```python
from build123d import *

# Parameters (mm, degrees)
BOSS_EXTRUDE1_DEPTH       = 12.7
SKETCH2_R                 = 5.635000033
HAPTIC_MOTOR_CUTOUT_DEPTH = 9.557999934
SKETCH3_W                 = 5.08
SKETCH3_H                 = 6.35
HAPTIC_WIRE_CUTOUT_DEPTH  = 13.7
SKETCH4_W                 = 6.096
SKETCH4_H                 = 2.54
PINS_DEPTH                = 5.08


with BuildPart() as part:
    # Sketch1 → Boss-Extrude1 (new body)
    with BuildSketch(Plane(origin=(0, 0, 0), x_dir=(1, 0, 0), z_dir=(0, 1, 0))):
        Polygon((0, 0), (19.05, 0), (12.7, 19.05), (19.05, 38.1), (0, 38.1), (-6.35, 19.05), align=None)
    extrude(amount=BOSS_EXTRUDE1_DEPTH)

    # Sketch2 → Haptic Motor Cutout (cut)
    with BuildSketch(Plane.XZ.offset(-12.7)):
        with Locations((2.54, -19.05)):
            Circle(SKETCH2_R)
    extrude(amount=HAPTIC_MOTOR_CUTOUT_DEPTH, mode=Mode.SUBTRACT)

    # Sketch3 → Haptic Wire Cutout (cut, through all)
    with BuildSketch(Plane.XZ):
        with Locations((2.54, -27.255072104)):
            Rectangle(SKETCH3_W, SKETCH3_H)
    extrude(amount=-HAPTIC_WIRE_CUTOUT_DEPTH, mode=Mode.SUBTRACT)

    # Sketch4 → Pins (add)
    with BuildSketch(Plane.XZ):
        with Locations((10.668, -35.56)):
            Rectangle(SKETCH4_W, SKETCH4_H)
    pins = extrude(amount=PINS_DEPTH)

    # Mirror1: Pins across plane
    add(pins.mirror(Plane(origin=(0, 0, -19.05), x_dir=(1, 0, 0), z_dir=(0, 0, -1))))


solid = part.part
```
Can you work these out from the model? Positions are in its coordinate system, mm. A direction names the side the tool comes from. Coordinates: 2 decimals unless noted, no trailing zeros. Loops run counter-clockwise (first coordinate to the right, second up) from the corner with the lowest first, then second, coordinate; pieces in that order, holes last.
1) Thinking about a two-plate mould opening in Z: for faces 6 (the flat face through (15.83, 6.26, -28.44)), 7 (the flat face through (9, 6, 0)), 8 (the flat face through (13.716, -3, -36)), which applies, pulls with the +Z half, pulls with the -Z half, needs draft (parallel to the pull), parting line crosses it, or undercut?
2) For pin 1 (4 mm diameter, centred on y = 0, z = -6.5, fed in from -X); pin 2 (2 mm diameter, centred on x = -2.5, z = -23, fed in from -Y); pin 3 (8.5 mm diameter, centred on x = 3.5, z = -20, fed in from +Y); pin 4 (5 mm diameter, centred on y = 9, z = -19.5, fed in from -X), each with a flat end and sliding along its axis, tell me the tip position at first contact or that it passes through.
3) Which directions (+Z, -Z, +X, -X, +Y, -Y) give clear straight access to the entire face, cutting with the end or side of a thin tool? Please do faces 1 (the flat face through (11, -3, -3.81)), 2 (the flat face through (11, -3, -36.83)), 3 (the flat face through (11, -3, -1.27)), 4 (the flat face through (5.08, 6, -27)), 5 (the flat face through (7.62, -3, -3)).
4) Imagine slicing it at B-B on y = 6. List the corners of the cut face in (x, z) for me (3 decimals), plus the area to 3 significant figures.
5) Imagine slicing it at C-C on y = -1.75. List the corners of the cut face in (x, z) for me, plus the area to 3 significant figures.
6) Imagine slicing it at D-D on x = 11.5. List the corners of the cut face in (y, z) for me, plus the area to 3 significant figures.
7) Imagine slicing it at A-A on x = 2.54. List the corners of the cut face in (y, z) for me (3 decimals), plus the area to 3 significant figures.
8) I need wall thicknesses on probe 1 along Z at (x, y) = (2.54, 10) (3 decimals); probe 2 along X at (y, z) = (10.75, -19.05) (3 decimals); probe 3 along Y at (x, z) = (14.5, -35). Which ranges of each line are inside material? Lowest first, please.
Completed:
1. face 6: undercut
1. face 7: pulls with the +Z half
1. face 8: needs draft
2. pin 1: stops at x = -2.83
2. pin 2: stops at y = 0
2. pin 3: stops at y = 3.14
2. pin 4: stops at x = -6.35
3. face 1: +X, -X, -Y
3. face 2: -Z, +X, -X, -Y
3. face 3: +Z, +X, -X, -Y
3. face 4: +Y, -Y
3. face 5: +Z, -Z, -X, -Y
4. outline: (-6.35, -19.05) - (0, -38.1) - (19.05, -38.1) - (12.7, -19.05) - (19.05, 0) - (0, 0) - close; hole (0, -30.43) - (5.08, -30.43) - (5.08, -24.08) arc R5.635 ccw (long way) to (0, -24.08) - close
4. area: 596 mm2
5. outline: (7.62, -36.83) - (13.72, -36.83) - (13.72, -34.29) - (7.62, -34.29) - close; (7.62, -3.81) - (13.72, -3.81) - (13.72, -1.27) - (7.62, -1.27) - close
5. area: 31.0 mm2
6. outline: (-5.08, -36.83) - (0, -36.83) - (0, -38.1) - (12.7, -38.1) - (12.7, 0) - (0, 0) - (0, -1.27) - (-5.08, -1.27) - (-5.08, -3.81) - (0, -3.81) - (0, -34.29) - (-5.08, -34.29) - close
6. area: 510 mm2
7. outline: (0, -38.1) - (12.7, -38.1) - (12.7, -30.43) - (0, -30.43) - close; (0, -24.08) - (3.142, -24.08) - (3.142, -13.415) - (12.7, -13.415) - (12.7, 0) - (0, 0) - close
7. area: 301 mm2
8. probe 1: z = -38.1 to -30.43, -13.415 to 0
8. probe 2: x = -6.35 to -3.095, 8.175 to 12.7
8. probe 3: y = 0 to 12.7
